from build123d import *

# Parameters (mm, degrees)
SKETCH1_W           = 30.5
SKETCH1_H           = 9.5
SKETCH1_W_2         = 29.5
SKETCH1_H_2         = 8.5
BOSS_EXTRUDE1_DEPTH = 20
BOSS_EXTRUDE2_DEPTH = 30.5
CUT_EXTRUDE1_DEPTH  = 1.5


with BuildPart() as part:
    # Sketch1 → Boss-Extrude1 (new body)
    with BuildSketch(Plane(origin=(0, 0, 0), x_dir=(1, 0, 0), z_dir=(0, 1, 0))):
        Rectangle(SKETCH1_W, SKETCH1_H)
        Rectangle(SKETCH1_W_2, SKETCH1_H_2, mode=Mode.SUBTRACT)
    extrude(amount=BOSS_EXTRUDE1_DEPTH)

    # Sketch2 → Boss-Extrude2 (add)
    with BuildSketch(Plane.ZY.offset(15.25)):
        Polygon((6.75, 18.147346039), (6.75, 0), (9.853378947, 17.600136599), align=None)
        Polygon((4.75, 18.5), (4.75, 0), (6.75, 0), (6.75, 18.147346039), align=None)
        Polygon((-6.5, 1.75), (-4.75, 20), (-4.75, 0), (-6.5, 0), align=None)
    extrude(amount=-BOSS_EXTRUDE2_DEPTH)

    # Sketch3 → Cut-Extrude1 (cut)
    with BuildSketch(Plane.ZY.offset(15.25)):
        Polygon((4.75, 18.5), (9.853378947, 17.600136599), (6.75, 0), (4.75, 0), align=None)
    cut_extrude1 = extrude(amount=-CUT_EXTRUDE1_DEPTH, mode=Mode.SUBTRACT)

    # Mirror1: Cut-Extrude1 across plane
    add(cut_extrude1.mirror(Plane.ZY), mode=Mode.SUBTRACT)


solid = part.part
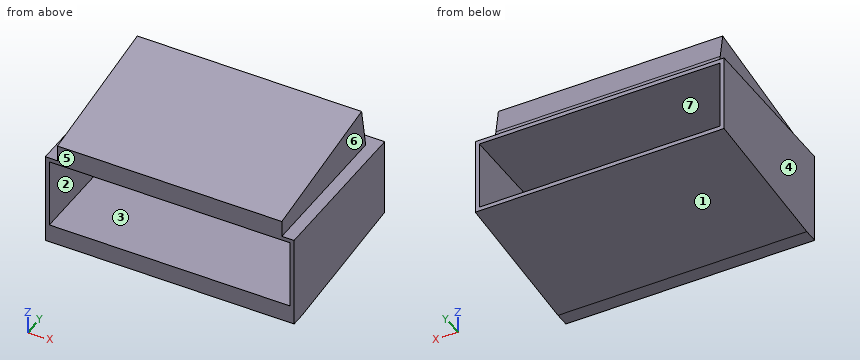
Input: part model. Units: mm. Frame: model coordinates. Face numbers are marked on the shaded views. A direction names the side the tool comes from. Give positions to 0.01 mm unless a question says otherwise; leave off trailing zeros. Loops run counter-clockwise (first coordinate to the right, second up) from the corner with the lowest first, then second, coordinate; pieces in that order, holes last. Notation, with made-up numbers: (44.5, -17) -> (49.5, -17) arc R25 cw to (49.5, 12) -> close; hole circle Ø4 at (-31, 23.25). An arc over 180 degrees is marked (long way). Answer as a JSON object with one key per item and string values. Group by question number.
Item 1: Pull-direction query (X, two-part tool) for the marked faces 1, 2, 3 and 4; classes: released by +X, released by -X, zero draft, split by the parting line, or undercut.
Item 2: Reachability of the marked faces 5, 6 and 7 from +Z, -Z, +X, -X, +Y, -Y: full face, straight path, thin tool, end or side. Return the list, or none.
Item 3: Cut plane C-C, the plane y = 4.25. Return the cut outline in (x, z).
Item 4: Cut plane D-D, the plane y = 12.5. Return the cut outline in (x, z).
Item 5: Pin query (flat end, axial travel): P1, Ø2, axis at x = 2, y = 10, coming from the -Z side; P2, Ø8, axis at x = -12, y = 11, coming from the +Z side; P3, Ø5, axis at x = -9, z = -3.5, coming from the +Y side; P4, Ø1, axis at x = -0.5, y = 5.5, coming from the -Z side. Return the tip coordinate at first contact, or that it passes through.
Item 6: Cut plane B-B, the plane z = -3.5. Return the cut outline in (x, y), and give its area (3 significant figures).
Item 7: Line query: probe 1 along X at (y, z) = (12, -1.75); probe 2 along Z at (x, y) = (-12, 7.75); probe 3 along Z at (x, y) = (0.5, 18.75). Output: solid intervals per line, ascending.
Item 8: Cut plane A-A, the plane x = 8. Return the cut outline in (y, z).
Checks:
{
 "1": {"face 1": "zero draft", "face 2": "undercut", "face 3": "undercut", "face 4": "released by -X"},
 "2": {"face 5": "+Z, -Z, +X, -X, -Y", "face 6": "+Z, +X, +Y, -Y", "face 7": "+Y, -Y"},
 "3": {"outline": "(-15.25, -6.26) -> (15.25, -6.26) -> (15.25, 4.75) -> (13.75, 4.75) -> (13.75, 7.5) -> (-13.75, 7.5) -> (-13.75, 4.75) -> (-15.25, 4.75) -> close; hole (-14.75, -4.25) -> (14.75, -4.25) -> (14.75, 4.25) -> (-14.75, 4.25) -> close"},
 "4": {"outline": "(-15.25, -5.47) -> (15.25, -5.47) -> (15.25, 4.75) -> (13.75, 4.75) -> (13.75, 8.95) -> (-13.75, 8.95) -> (-13.75, 4.75) -> (-15.25, 4.75) -> close; hole (-14.75, -4.25) -> (14.75, -4.25) -> (14.75, 4.25) -> (-14.75, 4.25) -> close"},
 "5": {"P1": "stops at z = -5.8", "P2": "stops at z = 9.39", "P3": "stops at y = 20", "P4": "stops at z = -6.19"},
 "6": {"outline": "(-15.25, 0) -> (-14.75, 0) -> (-14.75, 20) -> (-15.25, 20) -> close; (14.75, 0) -> (15.25, 0) -> (15.25, 20) -> (14.75, 20) -> close", "area": "20.0 mm²"},
 "7": {"probe 1": "x = -15.25 to -14.75, 14.75 to 15.25", "probe 2": "z = -5.92 to -4.25, 4.25 to 8.12", "probe 3": "z = -4.87 to -4.25, 4.25 to 4.75"},
 "8": {"outline": "(0, -6.5) -> (1.75, -6.5) -> (20, -4.75) -> (20, -4.25) -> (0, -4.25) -> close; (0, 4.25) -> (20, 4.25) -> (20, 4.75) -> (18.5, 4.75) -> (17.6, 9.85) -> (0, 6.75) -> close"}
}
